Source: CAD feature listing. Evaluate the final solid. Frame: model axes, mm. A direction names the side the tool comes from. Give positions to 0.01 mm unless a question says otherwise; leave off trailing zeros. Put each result on its own line as item: value.
```python
from build123d import *

# Parameters (mm, degrees)
F0_W     = 120.6359267235
F0_H     = 49.3188030086
F0_W_2   = 3.5166996237
F0_H_2   = 32.9512721967
F1_DEPTH = 9.144


with BuildPart() as f1:
    # F0 (on Front) → F1 (new body)
    with BuildSketch(Plane.XZ):
        with Locations((2.8384923935, 21.9962981064)):
            Rectangle(F0_W, F0_H)
        with BuildLine():
            add(Edge.make_bspline(
                [(-3.5570494323, 27.3089231075), (-0.687449643, 24.0666480209), (-0.687449643, 18.5442777062)],
                knots=[0, 0, 0, 1, 1, 1], degree=2))
            add(Edge.make_bspline(
                [(-0.687449643, 18.5442777062), (-0.687449643, 12.8660613581), (-3.5434976033, 9.6779935875)],
                knots=[0, 0, 0, 1, 1, 1], degree=2))
            add(Edge.make_bspline(
                [(-3.5434976033, 9.6779935875), (-6.3995455636, 6.4899258168), (-11.440825949, 6.4899258168)],
                knots=[0, 0, 0, 1, 1, 1], degree=2))
            add(Edge.make_bspline(
                [(-11.440825949, 6.4899258168), (-14.5577466175, 6.4899258168), (-16.9699721782, 7.9535233481)],
                knots=[0, 0, 0, 1, 1, 1], degree=2))
            add(Edge.make_bspline(
                [(-16.9699721782, 7.9535233481), (-19.382197739, 9.4171208793), (-20.6967251513, 12.1478144214)],
                knots=[0, 0, 0, 1, 1, 1], degree=2))
            add(Edge.make_bspline(
                [(-20.6967251513, 12.1478144214), (-22.0112525637, 14.8785079636), (-22.0112525637, 18.5442777062)],
                knots=[0, 0, 0, 1, 1, 1], degree=2))
            add(Edge.make_bspline(
                [(-22.0112525637, 18.5442777062), (-22.0112525637, 24.2157181398), (-19.1721443896, 27.3834581669)],
                knots=[0, 0, 0, 1, 1, 1], degree=2))
            add(Edge.make_bspline(
                [(-19.1721443896, 27.3834581669), (-16.3330362156, 30.5511981941), (-11.2917558301, 30.5511981941)],
                knots=[0, 0, 0, 1, 1, 1], degree=2))
            add(Edge.make_bspline(
                [(-11.2917558301, 30.5511981941), (-6.4266492216, 30.5511981941), (-3.5570494323, 27.3089231075)],
                knots=[0, 0, 0, 1, 1, 1], degree=2))
        make_face(mode=Mode.SUBTRACT)
        with BuildLine():
            Line((33.3276411297, 6.9168084301), (30.7189140485, 6.9168084301))
            Line((30.7189140485, 6.9168084301), (30.0209948554, 10.2234547044))
            Line((30.0209948554, 10.2234547044), (29.851596993, 10.2234547044))
            add(Edge.make_bspline(
                [(29.851596993, 10.2234547044), (28.1169628818, 8.0416102365), (26.3924926425, 7.2657680267)],
                knots=[0, 0, 0, 1, 1, 1], degree=2))
            add(Edge.make_bspline(
                [(26.3924926425, 7.2657680267), (24.6680224031, 6.4899258168), (22.0796230654, 6.4899258168)],
                knots=[0, 0, 0, 1, 1, 1], degree=2))
            add(Edge.make_bspline(
                [(22.0796230654, 6.4899258168), (18.6306825867, 6.4899258168), (16.6724432972, 8.2719913294)],
                knots=[0, 0, 0, 1, 1, 1], degree=2))
            add(Edge.make_bspline(
                [(16.6724432972, 8.2719913294), (14.7142040077, 10.054056842), (14.7142040077, 13.3335994583)],
                knots=[0, 0, 0, 1, 1, 1], degree=2))
            add(Edge.make_bspline(
                [(14.7142040077, 13.3335994583), (14.7142040077, 20.3602227913), (25.9554461574, 20.6990185161)],
                knots=[0, 0, 0, 1, 1, 1], degree=2))
            Line((25.9554461574, 20.6990185161), (29.8922524799, 20.8277608915))
            Line((29.8922524799, 20.8277608915), (29.8922524799, 22.2710306793))
            add(Edge.make_bspline(
                [(29.8922524799, 22.2710306793), (29.8922524799, 25.0017242214), (28.720019272, 26.3026998047)],
                knots=[0, 0, 0, 1, 1, 1], degree=2))
            add(Edge.make_bspline(
                [(28.720019272, 26.3026998047), (27.5477860641, 27.6036753881), (24.9593867264, 27.6036753881)],
                knots=[0, 0, 0, 1, 1, 1], degree=2))
            add(Edge.make_bspline(
                [(24.9593867264, 27.6036753881), (22.0592953219, 27.6036753881), (18.4003014938, 25.82838579)],
                knots=[0, 0, 0, 1, 1, 1], degree=2))
            Line((18.4003014938, 25.82838579), (17.3161551743, 28.5184238451))
            add(Edge.make_bspline(
                [(17.3161551743, 28.5184238451), (19.030461542, 29.4467241311), (21.0733997627, 29.9752454619)],
                knots=[0, 0, 0, 1, 1, 1], degree=2))
            add(Edge.make_bspline(
                [(21.0733997627, 29.9752454619), (23.1163379834, 30.5037667926), (25.1762159903, 30.5037667926)],
                knots=[0, 0, 0, 1, 1, 1], degree=2))
            add(Edge.make_bspline(
                [(25.1762159903, 30.5037667926), (29.3230756622, 30.5037667926), (31.325358396, 28.6641060068)],
                knots=[0, 0, 0, 1, 1, 1], degree=2))
            add(Edge.make_bspline(
                [(31.325358396, 28.6641060068), (33.3276411297, 26.824445221), (33.3276411297, 22.7588965231)],
                knots=[0, 0, 0, 1, 1, 1], degree=2))
            Line((33.3276411297, 22.7588965231), (33.3276411297, 6.9168084301))
        make_face(mode=Mode.SUBTRACT)
        with BuildLine():
            Line((59.9637610157, 6.9168084301), (56.4470613919, 6.9168084301))
            Line((56.4470613919, 6.9168084301), (56.4470613919, 21.9322349545))
            add(Edge.make_bspline(
                [(56.4470613919, 21.9322349545), (56.4470613919, 24.764567214), (55.1562496803, 26.1637935576)],
                knots=[0, 0, 0, 1, 1, 1], degree=2))
            add(Edge.make_bspline(
                [(55.1562496803, 26.1637935576), (53.8654379688, 27.5630199011), (51.1076407687, 27.5630199011)],
                knots=[0, 0, 0, 1, 1, 1], degree=2))
            add(Edge.make_bspline(
                [(51.1076407687, 27.5630199011), (47.468974684, 27.5630199011), (45.7749960599, 25.5946167399)],
                knots=[0, 0, 0, 1, 1, 1], degree=2))
            add(Edge.make_bspline(
                [(45.7749960599, 25.5946167399), (44.0810174357, 23.6262135786), (44.0810174357, 19.0931267804)],
                knots=[0, 0, 0, 1, 1, 1], degree=2))
            Line((44.0810174357, 19.0931267804), (44.0810174357, 6.9168084301))
            Line((44.0810174357, 6.9168084301), (40.564317812, 6.9168084301))
            Line((40.564317812, 6.9168084301), (40.564317812, 30.1243155808))
            Line((40.564317812, 30.1243155808), (43.4237537296, 30.1243155808))
            Line((43.4237537296, 30.1243155808), (43.9929305473, 26.9464116819))
            Line((43.9929305473, 26.9464116819), (44.1623284097, 26.9464116819))
            add(Edge.make_bspline(
                [(44.1623284097, 26.9464116819), (45.2464747291, 28.6607180495), (47.1945501469, 29.6059581218)],
                knots=[0, 0, 0, 1, 1, 1], degree=2))
            add(Edge.make_bspline(
                [(47.1945501469, 29.6059581218), (49.1426255647, 30.5511981941), (51.5345233819, 30.5511981941)],
                knots=[0, 0, 0, 1, 1, 1], degree=2))
            add(Edge.make_bspline(
                [(51.5345233819, 30.5511981941), (55.7288144553, 30.5511981941), (57.8462877355, 28.5285877169)],
                knots=[0, 0, 0, 1, 1, 1], degree=2))
            add(Edge.make_bspline(
                [(57.8462877355, 28.5285877169), (59.9637610157, 26.5059772396), (59.9637610157, 22.0542014154)],
                knots=[0, 0, 0, 1, 1, 1], degree=2))
            Line((59.9637610157, 22.0542014154), (59.9637610157, 6.9168084301))
        make_face(mode=Mode.SUBTRACT)
        with BuildLine():
            add(Edge.make_bspline(
                [(-31.0943659463, 33.8747842546), (-27.0931884361, 29.8736067444), (-27.0931884361, 22.6911373781)],
                knots=[0, 0, 0, 1, 1, 1], degree=2))
            add(Edge.make_bspline(
                [(-27.0931884361, 22.6911373781), (-27.0931884361, 15.0275780825), (-31.253599937, 10.9721932563)],
                knots=[0, 0, 0, 1, 1, 1], degree=2))
            add(Edge.make_bspline(
                [(-31.253599937, 10.9721932563), (-35.4140114379, 6.9168084301), (-43.2266408524, 6.9168084301)],
                knots=[0, 0, 0, 1, 1, 1], degree=2))
            Line((-43.2266408524, 6.9168084301), (-51.804948605, 6.9168084301))
            Line((-51.804948605, 6.9168084301), (-51.804948605, 37.8759617649))
            Line((-51.804948605, 37.8759617649), (-42.3186683098, 37.8759617649))
            add(Edge.make_bspline(
                [(-42.3186683098, 37.8759617649), (-35.0955434565, 37.8759617649), (-31.0943659463, 33.8747842546)],
                knots=[0, 0, 0, 1, 1, 1], degree=2))
        make_face(mode=Mode.SUBTRACT)
        with Locations((7.2369823607, 23.3924445285)):
            Rectangle(F0_W_2, F0_H_2, mode=Mode.SUBTRACT)
    extrude(amount=F1_DEPTH)


solid = f1.part
```
(1) Line query: probe 1 along X at (y, z) = (-3.5, 31); probe 2 along Z at (x, y) = (28.5, -2.5); probe 3 along X at (y, z) = (-1, 32.5). Output: solid intervals per line, ascending. Write a range as from..to.
Calculated:
probe 1: x = -57.48..-51.8, -28.95..5.48, 9..63.16
probe 2: z = -2.66..8.74, 20.78..26.52, 30.12..46.66
probe 3: x = -57.48..-51.8, -29.91..5.48, 9..63.16
(2) Draft query along Z for faces 3 (the flat face through (2, -5, 46.656)), 4 (the flat face through (17.866, -4.508, 27.155)), 5 (the flat face through (2, 0, 22)). Return one class per face: released by +Z, released by -Z, zero draft, split by the parting line, or undercut.
Calculated:
face 3: released by +Z
face 4: undercut
face 5: zero draft
(3) Reachability of faces 1 (the flat face through (59.964, -5, 15)), 2 (the flat face through (2, -5, -2.663)) from +Z, -Z, +X, -X, +Y, -Y: full face, straight path, thin tool, end or side. Return the list, or none.
Calculated:
face 1: +Y, -Y
face 2: -Z, +X, -X, +Y, -Y
(4) Section A-A on y = -3. Give the number of separate pieces and of enclosed holes in the cut face, then the cut area to 3 significant figures.
Calculated:
separate pieces: 1
enclosed holes: 5
area: 4,250 mm²
